Build history of the part. All positions in model axes, mm. Face numbers are marked on the shaded views. Give positions to 0.01 mm unless a question says otherwise; leave off trailing zeros. Loops run counter-clockwise (first coordinate to the right, second up) from the corner with the lowest first, then second, coordinate; pieces in that order, holes last.
1) Two-plate mould, pull along X, no slides. Class the marked faces 1, 2 and 3: +X half, -X half, draft (parallel to the pull), parting line (faces both ways), or undercut.
2) Band-saw the part on C-C on x = 4.5. List the corners of the cut face in (y, z) (3 decimals).
3) Wall check: line 1 (Y direction, x = 15.5, z = 9.25); line 2 (X direction, y = 2, z = 2.75); line 3 (X direction, y = -3.5, z = 1.5). Give the ranges that are in metal, low to high.
4) Band-saw the part on D-D on x = -16. List the corners of the cut face in (y, z) (3 decimals), then the cut area to 3 significant figures.
5) Band-saw the part on B-B on y = 0. List the corners of the cut face in (x, z) (1 decimal), then the cut area to 3 significant figures.
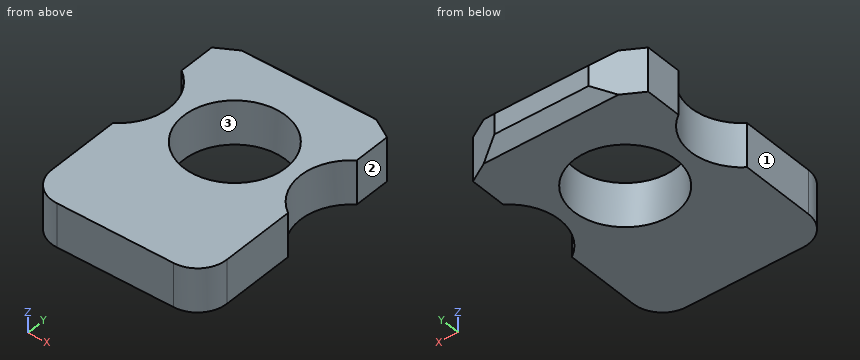
```python
from build123d import *

# Parameters (mm, degrees)
F0_R       = 11.1125
F1_DEPTH   = 9.525
F2_SIZE2   = 8.7988181024
F2_SIZE    = 5.08
F2_2_SIZE2 = 8.7988181024
F2_2_SIZE  = 5.08
F3_SIZE2   = 2.54
F3_SIZE    = 2.54
F4_R       = 6.35


with BuildPart() as f1:
    # F0 (on Top) → F1 (new body)
    with BuildSketch(Plane.XY):
        with BuildLine():
            Line((19.05, 22.225), (-19.05, 22.225))
            Line((-19.05, 22.225), (-19.05, 9.1194932014))
            ThreePointArc((-19.05, 9.1194932014), (-14.2875, 0), (-19.05, -9.1194932014))
            Line((-19.05, -9.1194932014), (-19.05, -31.75))
            Line((-19.05, -31.75), (19.05, -31.75))
            Line((19.05, -31.75), (19.05, -9.1194932014))
            ThreePointArc((19.05, -9.1194932014), (14.2875, 0), (19.05, 9.1194932014))
            Line((19.05, 9.1194932014), (19.05, 22.225))
        make_face()
        Circle(F0_R, mode=Mode.SUBTRACT)
    extrude(amount=F1_DEPTH)

    # F2
    f2_edges = [f1.edges().sort_by_distance(p)[0] for p in [
        (-19.05, 22.225, 4.7625),
    ]]
    f2_side = f1.faces().sort_by_distance((-19.05, 15.672247, 4.7625))[0]
    chamfer(f2_edges, length=F2_SIZE, length2=F2_SIZE2, reference=f2_side)

    # F2#2
    f2_2_edges = [f1.edges().sort_by_distance(p)[0] for p in [
        (19.05, 22.225, 4.7625),
    ]]
    f2_2_side = f1.faces().sort_by_distance((19.05, 15.672247, 4.7625))[0]
    chamfer(f2_2_edges, length=F2_2_SIZE, length2=F2_2_SIZE2, reference=f2_2_side)

    # F3
    f3_edges = [f1.edges().sort_by_distance(p)[0] for p in [
        (0, 22.225, 9.525),
        (0, 22.225, 0),
    ]]
    chamfer(f3_edges, length=F3_SIZE, length2=F3_SIZE2)

    # F4
    f4_edges = [f1.edges().sort_by_distance(p)[0] for p in [
        (19.05, -31.75, 4.7625),
        (-19.05, -31.75, 4.7625),
    ]]
    fillet(f4_edges, radius=F4_R)


solid = f1.part
```
Findings below:
1. face 1: -X half
1. face 2: +X half
1. face 3: undercut
2. outline: (-31.75, 0) - (-10.161, 0) - (-10.161, 9.525) - (-31.75, 9.525) - close; (10.161, 0) - (19.685, 0) - (22.225, 2.54) - (22.225, 6.985) - (19.685, 9.525) - (10.161, 9.525) - close
3. line 1: y = -31.1 to -5.05, 5.05 to 19.19
3. line 2: x = -14.47 to -10.93, 10.93 to 14.47
3. line 3: x = -14.85 to -10.55, 10.55 to 14.85
4. outline: (-30.825, 0) - (-5.927, 0) - (-5.927, 9.525) - (-30.825, 9.525) - close; (5.927, 0) - (18.906, 0) - (18.906, 9.525) - (5.927, 9.525) - close
4. area: 361 mm2
5. outline: (-14.3, 0) - (-11.1, 0) - (-11.1, 9.5) - (-14.3, 9.5) - close; (11.1, 0) - (14.3, 0) - (14.3, 9.5) - (11.1, 9.5) - close
5. area: 60.5 mm2
